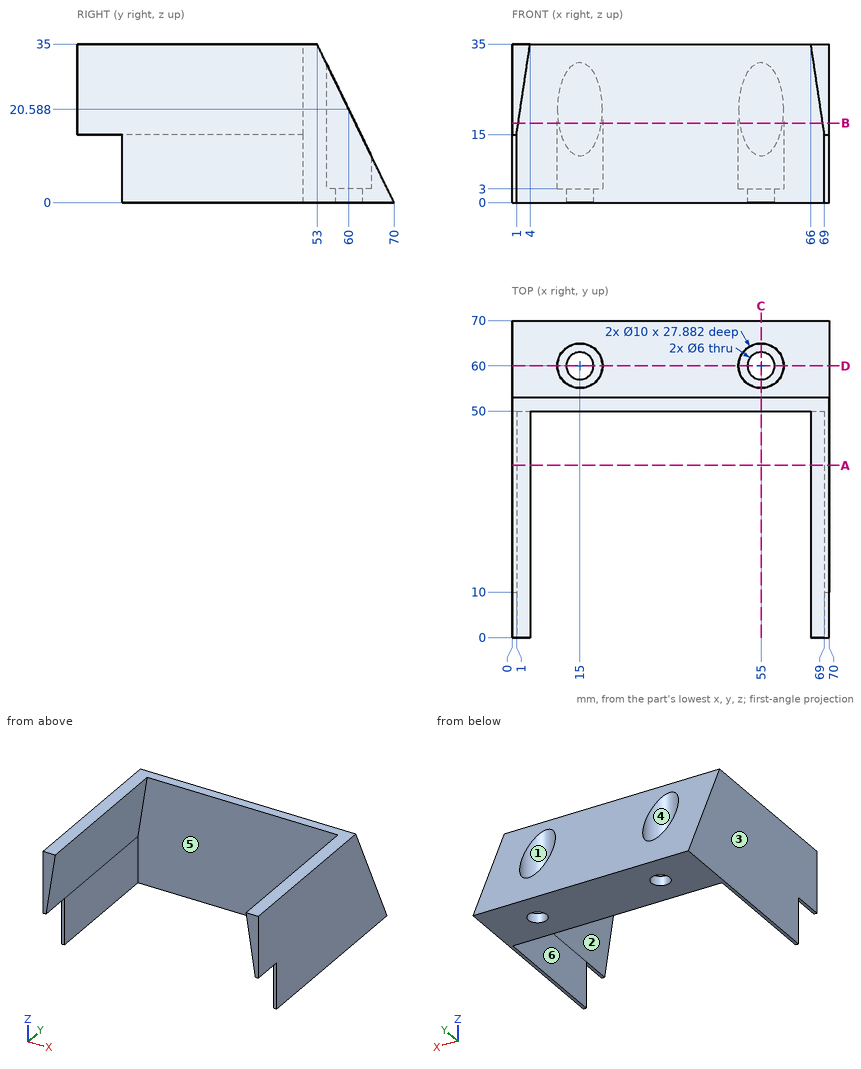
Geometry check sheet. Reference: drawing and pictorial views, mm from the part's lowest x, y, z. A direction names the side the tool comes from. Coordinates: 2 decimals unless noted, no trailing zeros. Order: outer loops, then holes, each group sorted by start corner. A loop starts at its lowest first (then second) coordinate and runs counter-clockwise, first axis right, second up. Notation, with made-up numbers: (8.5, 4.25) -> (54.5, 4.25) arc R28 ccw to (54.5, 29.25) -> close; hole circle Ø1 at (-34.75, 59). An arc over 180 degrees is marked (long way). Put each result on its own line as item: value. Start each with the question number.
1) Material ranges on L1, parallel to X at y = 60, z = 20.5; L2, parallel to X at y = 63, z = 13.5; L3, parallel to X at y = 34, z = 14.5, recorded low to high.
2) Go/stop test with flat-tipped pins: pin 1 (1 mm diameter, centred on x = 52.5, z = 7.5, fed in from -Y); pin 2 (11.5 mm diameter, centred on x = 55, y = 60, fed in from +Z) (1 decimal); pin 3 (5 mm diameter, centred on x = 7, z = 18.5, fed in from +Y). Record where each tip stops, or that it passes through.
3) Cross-section at A-A (y = 38). Enter the section's corners in (x, z), plus the area to 3 significant figures.
4) Tool access check on the marked faces 1, 2 and 3. Record the directions out of +Z, -Z, +X, -X, +Y, -Y that give a thin tool (end or side, any length) a straight path to the whole face; none if there is none.
5) Cross-section at C-C (x = 55). Enter the section's corners in (y, z), plus the area to 3 significant figures.
6) Cross-section at B-B (z = 17.5). Enter the section's corners in (x, y) (1 decimal).
7) Cross-section at D-D (y = 60). Enter the section's corners in (x, z).
8) Release check for a two-part mould opening along Y. For the marked faces 4, 5 and 6 record: pulls with the +Y half, pulls with the -Y half, needs draft (parallel to the pull), parting line crosses it, or undercut.
Geometry check:
1. L1: x = 0 to 10, 20 to 50, 60 to 70
1. L2: x = 0 to 11, 19 to 51, 59 to 70
1. L3: x = 0 to 1, 69 to 70
2. pin 1: stops at y = 50
2. pin 2: stops at z = 32.4
2. pin 3: stops at y = 62.23
3. outline: (0, 0) -> (1, 0) -> (1, 15) -> (4, 35) -> (0, 35) -> close; (66, 35) -> (69, 15) -> (69, 0) -> (70, 0) -> (70, 35) -> close
3. area: 130 mm^2
4. face 1: +Z
4. face 2: -Z, -Y
4. face 3: +Z, -Z, -X, +Y, -Y
5. outline: (50, 0) -> (57, 0) -> (57, 3) -> (55, 3) -> (55, 30.88) -> (53, 35) -> (50, 35) -> close; (63, 0) -> (70, 0) -> (65, 10.29) -> (65, 3) -> (63, 3) -> close
5. area: 209 mm^2
6. outline: (0, 0) -> (1.4, 0) -> (1.4, 50) -> (68.6, 50) -> (68.6, 0) -> (70, 0) -> (70, 61.5) -> (59.8, 61.5) arc R5 cw (long way) to (50.2, 61.5) -> (19.8, 61.5) arc R5 cw (long way) to (10.2, 61.5) -> (0, 61.5) -> close
7. outline: (0, 0) -> (12, 0) -> (12, 3) -> (10, 3) -> (10, 20.59) -> (0, 20.59) -> close; (18, 0) -> (52, 0) -> (52, 3) -> (50, 3) -> (50, 20.59) -> (20, 20.59) -> (20, 3) -> (18, 3) -> close; (58, 0) -> (70, 0) -> (70, 20.59) -> (60, 20.59) -> (60, 3) -> (58, 3) -> close
8. face 4: undercut
8. face 5: pulls with the -Y half
8. face 6: needs draft
